For this review, use the dimensioned drawing (mm, ordinates from the lowest corner) and the shaded views. A direction names the side the tool comes from. Coordinates: 2 decimals unless noted, no trailing zeros. Order: outer loops, then holes, each group sorted by start corner. A loop starts at its lowest first (then second) coordinate and runs counter-clockwise, first axis right, second up. Notation, with made-up numbers: M -3.5,62.5 L 12.5,62.5 A13 cw 12.5,70.5 Z; hole C -18.5,-28.5 d2. An arc over 180 degrees is marked long. Write each question's results on one line, items separated by ' | '.
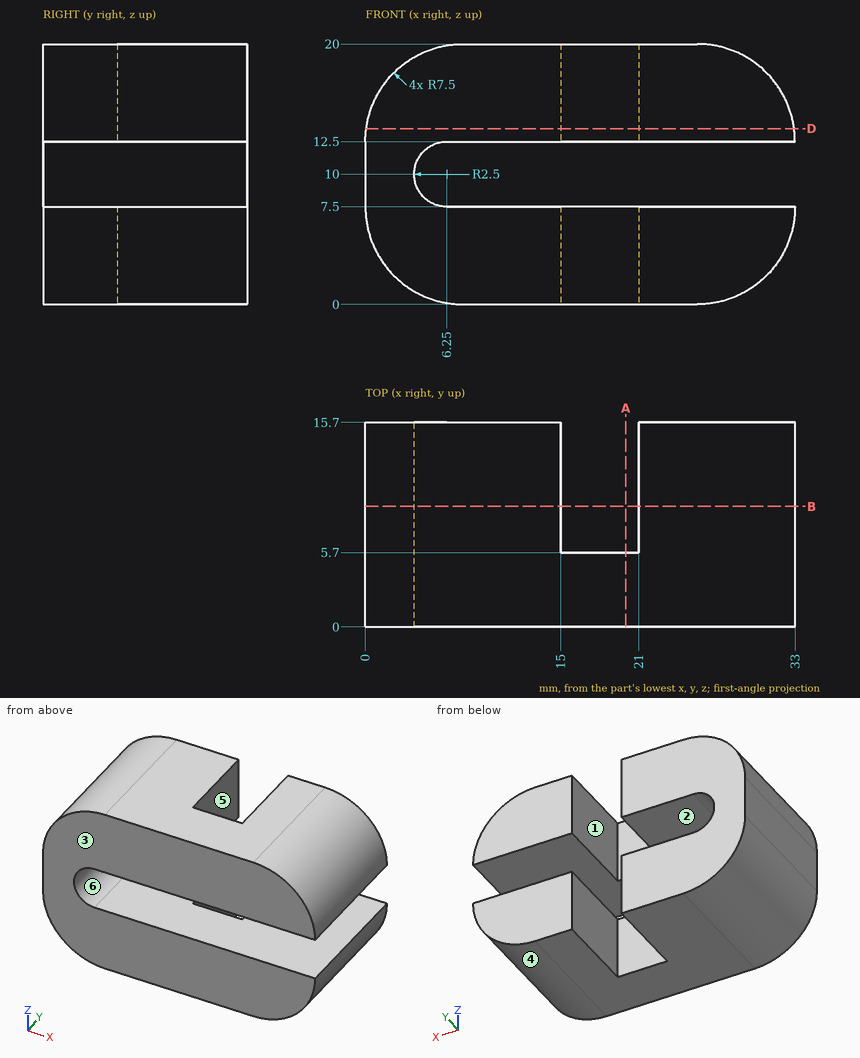
1) Take a section at A-A on x = 20. State the section outline as (y, z) points.
Solutions:
outline: M 0,0 L 5.7,0 L 5.7,7.5 L 0,7.5 Z; M 0,12.5 L 5.7,12.5 L 5.7,20 L 0,20 Z
2) The part is to be moulded in two halves that separate along Z. For the marked faces 4, 5 and 6, say which applies: pulls with the +Z half, pulls with the -Z half, needs draft (parallel to the pull), parting line crosses it, or undercut.
Solutions:
face 4: pulls with the -Z half | face 5: needs draft | face 6: undercut
3) For the marked faces 1, 2 and 3, list the 3-axis set-ups (+Z, -Z, +X, -X, +Y, -Y) from which the entire face can be reached by the end or side of a thin tool; tool diameter is ignored.
Solutions:
face 1: +Z, -Z, +Y | face 2: +X, +Y, -Y | face 3: +Z, -Z, +X, -X, -Y
4) Take a section at D-D on z = 13.5. State the section outline as (x, y) points, plus the area to 3 significant figures.
Solutions:
outline: M 0.07,0 L 32.93,0 L 32.93,15.7 L 21,15.7 L 21,5.7 L 15,5.7 L 15,15.7 L 0.07,15.7 Z | area: 456 mm2
5) To check wall thickness, follow line 1 along Z through (x, y) = (21.5, 7.5); line 2 along Y through (x, z) = (20.5, 18.5); line 3 along X through (y, z) = (15, 5.5). State the ranges of each line that lie inside material, in increasing order.
Solutions:
line 1: 0 to 7.5, 12.5 to 20 | line 2: 0 to 5.7 | line 3: 0.27 to 15, 21 to 32.73
6) Take a section at B-B on y = 9.25. Count the separate pieces of the cut face and the enclosed holes in it, plus the area to 3 significant figures.
Solutions:
separate pieces: 3 | enclosed holes: 0 | area: 378 mm2
7) For pin 1 (3 mm diameter, centred on y = 3, z = 8, fed in from +X); pin 2 (2 mm diameter, centred on x = 27, y = 2.5, fed in from +Z); pin 3 (6 mm diameter, centred on y = 12, z = 3, fed in from +X); pin 4 (4 mm diameter, centred on y = 12, z = 2, fed in from -X), all flat-tipped, find the tip position at first contact; note any pin that passes through.
Solutions:
pin 1: x = 33 | pin 2: z = 19.98 | pin 3: x = 32.85 | pin 4: x = 0.87
